CAD build for the part. Positions are in the model's coordinates, mm. Give positions to 0.01 mm unless a question says otherwise; leave off trailing zeros. Write each loop counter-clockwise with the first axis right and the second up, starting at its lowest first coordinate (ties: lowest second). Pieces come first, ordered by that corner, then holes. Notation, with made-up numbers: (79.25, 15) - (98.25, 15) arc R15 cw to (98.25, 33) - close; hole circle Ø9 at (57, -7). An arc over 180 degrees is marked (long way). Answer as a JSON object with one key per item and string values.
from build123d import *

# Parameters (mm, degrees)
F0_W     = 120
F0_H     = 160
F0_R     = 6.1
F1_DEPTH = 4


with BuildPart() as f1:
    # F0 (on Front) → F1 (new body)
    with BuildSketch(Plane.XZ):
        Rectangle(F0_W, F0_H)
        with Locations((-39.5, -60)):
            Circle(F0_R, mode=Mode.SUBTRACT)
        with Locations((-20.5, -60)):
            Circle(F0_R, mode=Mode.SUBTRACT)
        with Locations((-39.5, -30)):
            Circle(F0_R, mode=Mode.SUBTRACT)
        with Locations((-20.5, -30)):
            Circle(F0_R, mode=Mode.SUBTRACT)
        with Locations((20.5, -60)):
            Circle(F0_R, mode=Mode.SUBTRACT)
        with Locations((39.5, -60)):
            Circle(F0_R, mode=Mode.SUBTRACT)
        with Locations((20.5, -30)):
            Circle(F0_R, mode=Mode.SUBTRACT)
        with Locations((39.5, -30)):
            Circle(F0_R, mode=Mode.SUBTRACT)
        with Locations((-39.5, 0)):
            Circle(F0_R, mode=Mode.SUBTRACT)
        with Locations((-39.5, 30)):
            Circle(F0_R, mode=Mode.SUBTRACT)
        with Locations((-20.5, 0)):
            Circle(F0_R, mode=Mode.SUBTRACT)
        with Locations((-20.5, 30)):
            Circle(F0_R, mode=Mode.SUBTRACT)
        with Locations((-39.5, 60)):
            Circle(F0_R, mode=Mode.SUBTRACT)
        with Locations((-20.5, 60)):
            Circle(F0_R, mode=Mode.SUBTRACT)
        with Locations((20.5, 0)):
            Circle(F0_R, mode=Mode.SUBTRACT)
        with Locations((20.5, 30)):
            Circle(F0_R, mode=Mode.SUBTRACT)
        with Locations((39.5, 0)):
            Circle(F0_R, mode=Mode.SUBTRACT)
        with Locations((39.5, 30)):
            Circle(F0_R, mode=Mode.SUBTRACT)
        with Locations((20.5, 60)):
            Circle(F0_R, mode=Mode.SUBTRACT)
        with Locations((39.5, 60)):
            Circle(F0_R, mode=Mode.SUBTRACT)
    extrude(amount=-F1_DEPTH)


solid = f1.part
(1) Saw through at B-B, the plane y = 2.3. State how many separate pieces and enclosed holes the cut face has, and give its area (3 significant figures).
Answer key:
{"separate pieces": "1", "enclosed holes": "20", "area": "16,900 mm²"}
(2) Probe L1, parallel to Z at x = 39.5, y = 2.75; L2, parallel to Z at x = 22, y = 0.35; L3, parallel to X at y = 3.5, z = 32.5. List the from-to ranges inside material, lowest first. Write a range as [from, to].
Answer key:
{"L1": "z = [-80, -66.1], [-53.9, -36.1], [-23.9, -6.1], [6.1, 23.9], [36.1, 53.9], [66.1, 80]", "L2": "z = [-80, -65.91], [-54.09, -35.91], [-24.09, -5.91], [5.91, 24.09], [35.91, 54.09], [65.91, 80]", "L3": "x = [-60, -45.06], [-33.94, -26.06], [-14.94, 14.94], [26.06, 33.94], [45.06, 60]"}
(3) Saw through at A-A, the plane z = -60. Give the cut face in (x, y), and give its area (3 significant figures).
Answer key:
{"outline": "(-60, 0) - (-45.6, 0) - (-45.6, 4) - (-60, 4) - close; (-33.4, 0) - (-26.6, 0) - (-26.6, 4) - (-33.4, 4) - close; (-14.4, 0) - (14.4, 0) - (14.4, 4) - (-14.4, 4) - close; (26.6, 0) - (33.4, 0) - (33.4, 4) - (26.6, 4) - close; (45.6, 0) - (60, 0) - (60, 4) - (45.6, 4) - close", "area": "285 mm²"}
(4) Pull direction Z, two halves, no side cores. Call faces 1 (the face through (-1, 0, 1)), 2 (the face through (-33.68, 1.97, 31.83)): pulls with the +Z half, pulls with the -Z half, needs draft (parallel to the pull), parting line crosses it, or undercut.
Answer key:
{"face 1": "needs draft", "face 2": "undercut"}
(5) Saw through at D-D, the plane x = -38. Give the cut face in (y, z), and give its area (3 significant figures).
Answer key:
{"outline": "(0, -80) - (4, -80) - (4, -65.91) - (0, -65.91) - close; (0, -54.09) - (4, -54.09) - (4, -35.91) - (0, -35.91) - close; (0, -24.09) - (4, -24.09) - (4, -5.91) - (0, -5.91) - close; (0, 5.91) - (4, 5.91) - (4, 24.09) - (0, 24.09) - close; (0, 35.91) - (4, 35.91) - (4, 54.09) - (0, 54.09) - close; (0, 65.91) - (4, 65.91) - (4, 80) - (0, 80) - close", "area": "403 mm²"}
(6) Flat gauge pin, fed straight in: P1, Ø16, axis at x = -39.5, z = 60, coming from the -Y side. Where does the tip first touch, or does it go through?
Answer key:
{"P1": "stops at y = 0"}
(7) Saw through at C-C, the plane x = 20.5. Give the cut face in (y, z).
Answer key:
{"outline": "(0, -80) - (4, -80) - (4, -66.1) - (0, -66.1) - close; (0, -53.9) - (4, -53.9) - (4, -36.1) - (0, -36.1) - close; (0, -23.9) - (4, -23.9) - (4, -6.1) - (0, -6.1) - close; (0, 6.1) - (4, 6.1) - (4, 23.9) - (0, 23.9) - close; (0, 36.1) - (4, 36.1) - (4, 53.9) - (0, 53.9) - close; (0, 66.1) - (4, 66.1) - (4, 80) - (0, 80) - close"}
